```python
from build123d import *

# Parameters (mm, degrees)
EXTRUDE_1_DEPTH     = 45
EXTRUDE_2_DEPTH     = 3.5
CUT_EXTRUDE_1_REACH = 77.166
CUT_EXTRUDE_2_REACH = 79.942
FILLET_1_R          = 2


with BuildPart() as part:
    # 草图1 → 凸台-拉伸1 (new body)
    with BuildSketch(Plane(origin=(0, 0, 0), x_dir=(0, 0, -1), z_dir=(1, 0, 0))):
        Polygon((0, 0), (0, 45), (5, 45), (5, 0), (45, 0), (45, -5), (0, -5), align=None)
    extrude(amount=EXTRUDE_1_DEPTH)

    # 草图2 → 凸台-拉伸2 (add)
    with BuildSketch(Plane(origin=(45, 0, 0), x_dir=(0, 0, -1), z_dir=(1, 0, 0))):
        Polygon((45, 0), (45, 2.5), (38, 2.5), (7.5, 38), (7.5, 45), (5, 45), (5, 0), align=None)
    extrude_2 = extrude(amount=-EXTRUDE_2_DEPTH)

    # 镜向1: 凸台-拉伸2 across plane
    add(extrude_2.mirror(Plane(origin=(22.5, 0, 0), x_dir=(0, 0, 1), z_dir=(1, 0, 0))))

    # 草图4 → 切除-拉伸1 (cut, up to next)
    with BuildSketch(Plane(origin=(0, 0, -5), x_dir=(-1, 0, 0), z_dir=(0, 0, -1)), mode=Mode.PRIVATE) as cut_extrude_1_sk1:
        with BuildLine():
            Line((-18.25, 33), (-18.25, 11.5))
            ThreePointArc((-18.25, 11.5), (-22.5, 7.25), (-26.75, 11.5))
            Line((-26.75, 11.5), (-26.75, 33))
            ThreePointArc((-26.75, 33), (-22.5, 37.25), (-18.25, 33))
        make_face()
    cut_extrude_1_tool1 = extrude(cut_extrude_1_sk1.sketch, amount=-CUT_EXTRUDE_1_REACH, mode=Mode.PRIVATE) & part.part
    add(cut_extrude_1_tool1.solids().sort_by_distance((22.5, 22.25, -5))[0], mode=Mode.SUBTRACT)

    # 草图5 → 切除-拉伸2 (cut, up to next)
    with BuildSketch(Plane(origin=(0, 0, 0), x_dir=(1, 0, 0), z_dir=(0, 1, 0)), mode=Mode.PRIVATE) as cut_extrude_2_sk1:
        with BuildLine():
            Line((26.75, 37), (26.75, 15.5))
            ThreePointArc((26.75, 15.5), (22.5, 11.25), (18.25, 15.5))
            Line((18.25, 15.5), (18.25, 37))
            ThreePointArc((18.25, 37), (22.5, 41.25), (26.75, 37))
        make_face()
    cut_extrude_2_tool1 = extrude(cut_extrude_2_sk1.sketch, amount=-CUT_EXTRUDE_2_REACH, mode=Mode.PRIVATE) & part.part
    add(cut_extrude_2_tool1.solids().sort_by_distance((22.5, 0, -26.25))[0], mode=Mode.SUBTRACT)

    # 圆角1
    fillet_1_edges = [part.edges().sort_by_distance(p)[0] for p in [
        (43.25, 45, -7.5),
        (43.25, 38, -7.5),
        (43.25, 2.5, -38),
        (43.25, 2.5, -45),
        (1.75, 2.5, -45),
        (1.75, 2.5, -38),
        (1.75, 38, -7.5),
        (1.75, 45, -7.5),
    ]]
    fillet(fillet_1_edges, radius=FILLET_1_R)


solid = part.part
```
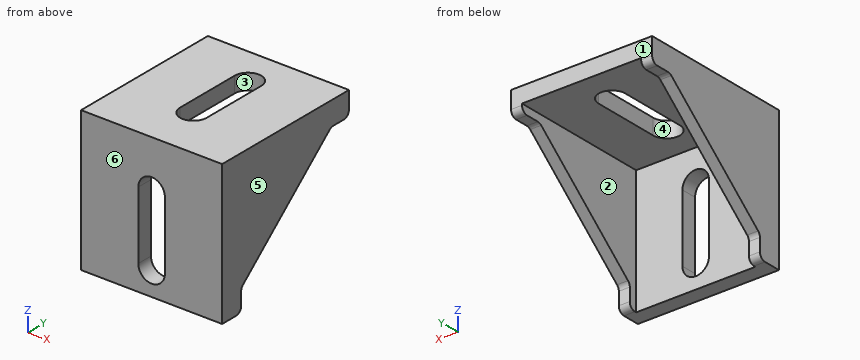
Check sheet for the modelled part. Datum: model origin and axes. Units: mm. Face numbers are marked on the shaded views. A direction names the side the tool comes from. Round coordinates to 2 decimals unless told otherwise and drop trailing zeros. Order: outer loops, then holes, each group sorted by start corner. A loop starts at its lowest first (then second) coordinate and runs counter-clockwise, first axis right, second up. Notation, with made-up numbers: (-38.5, 67) - (-25.5, 67) arc R38 cw to (-25.5, 105) - close; hole circle Ø11 at (80, -16). An arc over 180 degrees is marked (long way). Write item = value, one per line.
Q1. Thickness scan on line 1 along X through (y, z) = (8, -12); line 2 along Y through (x, z) = (40.5, -41). Record the ranges inside material, lowest first.
Computed:
line_1 = 0 to 3.5, 41.5 to 45
line_2 = -5 to 0
Q2. Section check A-A (x = 22.5). Record the boundary of the cut face in (y, z).
Computed:
outline = (-5, -45) - (0, -45) - (0, -41.25) - (-5, -41.25) - close; (-5, -11.25) - (0, -11.25) - (0, -5) - (7.25, -5) - (7.25, 0) - (-5, 0) - close; (37.25, -5) - (45, -5) - (45, 0) - (37.25, 0) - close
Q3. Section check B-B (y = 21.5). Record the boundary of the cut face in (x, z), and give its area (3 significant figures).
Computed:
outline = (0, -21.68) - (3.5, -21.68) - (3.5, -5) - (18.25, -5) - (18.25, 0) - (0, 0) - close; (26.75, -5) - (41.5, -5) - (41.5, -21.68) - (45, -21.68) - (45, 0) - (26.75, 0) - close
area = 299 mm^2
Q4. Draft check along X on the marked faces 4, 5 and 6. Enter one of: pulls with the +X half, pulls with the -X half, needs draft (parallel to the pull), parting line crosses it, or undercut.
Computed:
face_4 = undercut
face_5 = pulls with the +X half
face_6 = needs draft
Q5. Go/stop test with flat-tipped pins: pin 1 (4 mm diameter, centred on x = 44, y = 40, fed in from -Z); pin 2 (1.8 mm diameter, centred on x = 1, y = 41.5, fed in from -Z); pin 3 (1.8 mm diameter, centred on x = 43, z = -40.5, fed in from +Y); pin 4 (6 mm diameter, centred on x = 23.5, y = 33.5, fed in from +Z). Record where each tip stops, or that it passes through.
Computed:
pin_1 = -7.64
pin_2 = -7.5
pin_3 = 2.5
pin_4 = through
Q6. Section check C-C (z = -24.5). Record the boundary of the cut face in (x, y).
Computed:
outline = (0, -5) - (18.25, -5) - (18.25, 0) - (3.5, 0) - (3.5, 18.21) - (0, 18.21) - close; (26.75, -5) - (45, -5) - (45, 18.21) - (41.5, 18.21) - (41.5, 0) - (26.75, 0) - close
Q7. Tool access check on the marked faces 1, 2 and 3. Record the directions out of +Z, -Z, +X, -X, +Y, -Y that give a thin tool (end or side, any length) a straight path to the whole face; none if there is none.
Computed:
face_1 = +Z, -Z, +X, -X, +Y
face_2 = -Z, +Y
face_3 = +Z, -Z
Q8. Section check D-D (x = 31). Record the boundary of the cut face in (y, z), and give its area (3 significant figures).
Computed:
outline = (-5, -45) - (0, -45) - (0, -5) - (45, -5) - (45, 0) - (-5, 0) - close
area = 450 mm^2
